Source: CAD feature listing. Evaluate the final solid. Frame: model axes, mm. Give positions to 0.01 mm unless a question says otherwise; leave off trailing zeros. Use CSV: the item, a comma, the result in double quotes. Start each with the question number.
1. Pin query (flat end, axial travel): P1, Ø0.8, axis at y = -3.5, z = 2, coming from the +X side; P2, Ø2, axis at y = 2.5, z = -1, coming from the -X side; P3, Ø2, axis at x = 2.5, z = 1.5, coming from the -Y side; P4, Ø0.6, axis at y = 3.5, z = 2, coming from the -X side. Return the tip coordinate at first contact, or that it passes through.
2. Mould query, pull axis Y, two halves, no side actions, for faces 1 (the flat face through (0, 0, 2)), 2 (the flat face through (0, 0, 5)). Classes: released by +Y, released by -Y, zero draft, split by the parting line, or undercut.
3. Line query: line 1 along Y through (x, z) = (-1.5, 1.75); line 2 along Y through (x, z) = (1.75, 2.5) (3 decimals); line 3 along Z through (x, y) = (-3.75, -2.75). Output: solid intervals per line, ascending. Write a range as [from, to].
4. Section query A-A, the plane z = 1.25. State how many separate pieces and enclosed holes the cut face has, plus the area to 3 significant figures.
from build123d import *

# Parameters (mm, degrees)
F4_W      = 8.7
F4_H      = 5.75
F3_W      = 9.3
F3_H      = 6.35
F5_W      = 8.7
F5_H      = 5.75
F9_DEPTH  = 0.5
F12_W     = 1.5
F12_H     = 0.2
F14_W     = 0.6195948031
F14_H     = 4.0430515073
F15_DEPTH = 25
F20_W     = 1.304730963
F20_H     = 4.4884709641
F21_DEPTH = 25
F22_W     = 1.5146217346
F22_H     = 4.5125598554
F23_DEPTH = 25


with BuildPart() as f6:
    # F4 (on offset) → F6 section 0
    with BuildSketch(Plane.XY.offset(2)):
        Rectangle(F4_W, F4_H)
    # F3 (on offset) → F6 section 1
    with BuildSketch(Plane.XY.offset(3.5)):
        Rectangle(F3_W, F3_H)
    loft()

    # F3 (on offset) → F7 section 0
    with BuildSketch(Plane.XY.offset(3.5)):
        Rectangle(F3_W, F3_H)
    # F5 (on offset) → F7 section 1
    with BuildSketch(Plane.XY.offset(5)):
        Rectangle(F5_W, F5_H)
    loft()

    # F8 (on face) → F9 (cut)
    with BuildSketch(Plane.XY.offset(5)):
        with BuildLine():
            Line((-4.5071290817, 0.9109661553), (-4.5071290817, -0.9109661553))
            ThreePointArc((-4.5071290817, -0.9109661553), (-3.936739006, 0), (-4.5071290817, 0.9109661553))
        make_face()
    extrude(amount=-F9_DEPTH, mode=Mode.SUBTRACT)



with BuildPart() as f13:
    # F13: sweep along a path in F10
    with BuildLine(Plane.YZ) as f13_path:
        Line((-2.0310959943, 3.5), (-3.3000006297, 3.5))
        ThreePointArc((-3.3000006297, 3.5), (-3.6532733467, 3.3538338416), (-3.8, 3.0007935498))
        Line((-3.8, 3.0007935498), (-3.81, -3.3))
    # F12 (on line) → F13 (sweep)
    with BuildSketch(Plane(origin=(0, -0.0052470193, -3.3060385298), x_dir=(1, 0, 0), z_dir=(0, -0.0015870997, -0.9999987406))):
        with Locations((0, 3.8047577726)):
            Rectangle(F12_W, F12_H)
    sweep(path=f13_path.line)

    # F14 (on face) → F15 (cut)
    with BuildSketch(Plane(origin=(0, -3.9047528548, 0.0061972398), x_dir=(1, 0, 0), z_dir=(0, -0.9999987406, 0.0015870997))):
        with Locations((-0.4997974016, -2.0215257537)):
            Rectangle(F14_W, F14_H)
        with Locations((0.4997974016, -2.0215257537)):
            Rectangle(F14_W, F14_H)
    extrude(amount=-F15_DEPTH, mode=Mode.SUBTRACT)


with BuildPart() as f13_1:
    # F16: moved
    add(f13.part.moved(Location((-1.27, 0, 0))))


with BuildPart() as f17_1:
    # F17: copy of F13
    add(f13_1.part.moved(Location((2.54, 0, 0))))


with BuildPart() as f18_1:
    # F18: copy of F13
    add(f13_1.part.moved(Location((-2.54, 0, 0))))

    # F20 (on face) → F21 (cut)
    with BuildSketch(Plane(origin=(0, -3.9047528548, 0.0061972398), x_dir=(1, 0, 0), z_dir=(0, -0.9999987406, 0.0015870997))):
        with Locations((-4.6523654815, 1.4981951099)):
            Rectangle(F20_W, F20_H)
    extrude(amount=-F21_DEPTH, mode=Mode.SUBTRACT)


with BuildPart() as f19_1:
    # F19: copy of F17_1
    add(f17_1.part.moved(Location((2.54, 0, 0))))

    # F22 (on face) → F23 (cut)
    with BuildSketch(Plane(origin=(0, -3.9047528548, 0.0061972398), x_dir=(1, 0, 0), z_dir=(0, -0.9999987406, 0.0015870997))):
        with Locations((4.7573108673, 1.4692934928)):
            Rectangle(F22_W, F22_H)
    extrude(amount=-F23_DEPTH, mode=Mode.SUBTRACT)


with BuildPart() as f6_1:
    add(f6.part)

    add(f13_1.part)  # F24 merges F13

    add(f17_1.part)  # F24 merges F17_1

    add(f18_1.part)  # F24 merges F18_1

    add(f19_1.part)  # F24 merges F19_1
    # F24: F18_1, F13, F17_1, F19_1 across plane
    add(f18_1.part.mirror(Plane.XZ))
    add(f13_1.part.mirror(Plane.XZ))
    add(f17_1.part.mirror(Plane.XZ))
    add(f19_1.part.mirror(Plane.XZ))


solid = f6_1.part
Result set:
1,P1,"x = 4"
1,P2,"through"
1,P3,"y = -3.9"
1,P4,"x = -4"
2,face 1,"undercut"
2,face 2,"zero draft"
3,line 1,"[-3.9, -3.7], [3.7, 3.9]"
3,line 2,"[-3.901, -3.701], [-2.975, 2.975], [3.701, 3.901]"
3,line 3,"[2, 5]"
4,separate pieces,"8"
4,enclosed holes,"0"
4,area,"1.95 mm2"
